Build history of the part. All positions in model axes, mm. Face numbers are marked on the shaded views. Round coordinates to 2 decimals unless told otherwise and drop trailing zeros. Loops run counter-clockwise (first coordinate to the right, second up) from the corner with the lowest first, then second, coordinate; pieces in that order, holes last. Notation, with made-up numbers: M 0,-10.75 L 49,-10.75 A30 cw 49,12.25 Z; hole C 84,82 d7. An arc over 180 degrees is marked long. One line per item, written item: value.
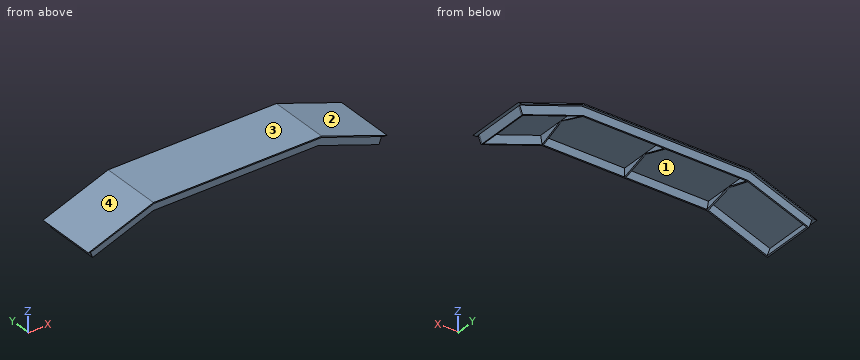
```python
from build123d import *

# Parameters (mm, degrees)
BOSS_EXTRUDE1_DEPTH = 109.600000002
BOSS_EXTRUDE2_DEPTH = 2.54
BOSS_EXTRUDE3_DEPTH = 2.54
RIB2_REACH          = 442.308
SKETCH5_WALL_W      = 932.745237508
SKETCH5_WALL_H      = 2.54
RIB3_REACH          = 442.308
SKETCH6_WALL_W      = 932.745237508
SKETCH6_WALL_H      = 2.54
RIB4_REACH          = 442.308
SKETCH7_WALL_W      = 932.745237508
SKETCH7_WALL_H      = 2.54
RIB5_REACH          = 442.308
SKETCH8_WALL_W      = 932.745237508
SKETCH8_WALL_H      = 2.54
RIB6_REACH          = 332.895
SKETCH13_WALL_W     = 713.849927416
SKETCH13_WALL_H     = 2.54
RIB7_REACH          = 332.895
SKETCH14_WALL_W     = 713.849927416
SKETCH14_WALL_H     = 2.54
SKETCH15_W          = 2.54
SKETCH15_H          = 95.520000222
BOSS_EXTRUDE4_DEPTH = 15
SKETCH16_W          = 2.54
SKETCH16_H          = 95.520000222
BOSS_EXTRUDE5_DEPTH = 15


with BuildPart() as part:
    # Sketch1 → Boss-Extrude1 (new body)
    with BuildSketch(Plane(origin=(0, 0, 0), x_dir=(1, 0, 0), z_dir=(0, 1, 0))):
        Polygon((-261, -120), (-150, -160), (150, -160), (261, -120), (266.899364373, -120), (150.349364373, -162), (-150.349364373, -162), (-266.899364373, -120), align=None)
    extrude(amount=BOSS_EXTRUDE1_DEPTH)

    # Sketch2 → Boss-Extrude2 (add)
    with BuildSketch(Plane(origin=(0, 4.49999989, 0), x_dir=(1, 0, 0), z_dir=(0, 1, 0))):
        Polygon((147.379767206, -145), (255.914706381, -105.888310207), (261, -120), (150, -160), (-150, -160), (-261, -120), (-255.914706381, -105.888310207), (-147.379767206, -145), align=None)
    extrude(amount=BOSS_EXTRUDE2_DEPTH)

    # Sketch4 → Boss-Extrude3 (add)
    with BuildSketch(Plane(origin=(0, 105.100000112, 0), x_dir=(1, 0, 0), z_dir=(0, 1, 0))):
        Polygon((-255.914706381, -105.888310207), (-147.379767206, -145), (147.379767206, -145), (255.914706381, -105.888310207), (261, -120), (150, -160), (-150, -160), (-261, -120), align=None)
    extrude(amount=-BOSS_EXTRUDE3_DEPTH)

    # Sketch5 wall → Rib2 (add, up to next)
    with BuildSketch(Plane(origin=(-148.689883603, 78.680000057, 152.5), x_dir=(-0.052270147277, -0.952748261703, 0.299229980995), z_dir=(0.163945637159, -0.303761007739, -0.938536668561)), mode=Mode.PRIVATE) as rib2_sk1:
        Rectangle(SKETCH5_WALL_W, SKETCH5_WALL_H)
    rib2_tool1 = extrude(rib2_sk1.sketch, amount=-RIB2_REACH, mode=Mode.PRIVATE) - part.part
    add(rib2_tool1.solids().sort_by_distance((-148.689883603, 78.680000057, 152.5))[0])

    # Sketch6 wall → Rib3 (add, up to next)
    with BuildSketch(Plane(origin=(-148.689883603, 30.919999945, 152.5), x_dir=(0.052270147277, -0.952748261703, -0.299229980995), z_dir=(0.163945637159, 0.303761007739, -0.938536668561)), mode=Mode.PRIVATE) as rib3_sk1:
        Rectangle(SKETCH6_WALL_W, SKETCH6_WALL_H)
    rib3_tool1 = extrude(rib3_sk1.sketch, amount=-RIB3_REACH, mode=Mode.PRIVATE) - part.part
    add(rib3_tool1.solids().sort_by_distance((-148.689883603, 30.919999945, 152.5))[0])

    # Sketch7 wall → Rib4 (add, up to next)
    with BuildSketch(Plane(origin=(148.689883603, 78.680000057, 152.5), x_dir=(0.052270147277, -0.952748261703, 0.299229980995), z_dir=(-0.163945637159, -0.303761007739, -0.938536668561)), mode=Mode.PRIVATE) as rib4_sk1:
        Rectangle(SKETCH7_WALL_W, SKETCH7_WALL_H)
    rib4_tool1 = extrude(rib4_sk1.sketch, amount=-RIB4_REACH, mode=Mode.PRIVATE) - part.part
    add(rib4_tool1.solids().sort_by_distance((148.689883603, 78.680000057, 152.5))[0])

    # Sketch8 wall → Rib5 (add, up to next)
    with BuildSketch(Plane(origin=(148.689883603, 30.919999945, 152.5), x_dir=(-0.052270147277, -0.952748261703, -0.299229980995), z_dir=(-0.163945637159, 0.303761007739, -0.938536668561)), mode=Mode.PRIVATE) as rib5_sk1:
        Rectangle(SKETCH8_WALL_W, SKETCH8_WALL_H)
    rib5_tool1 = extrude(rib5_sk1.sketch, amount=-RIB5_REACH, mode=Mode.PRIVATE) - part.part
    add(rib5_tool1.solids().sort_by_distance((148.689883603, 30.919999945, 152.5))[0])

    # Sketch13 wall → Rib6 (add, up to next)
    with BuildSketch(Plane(origin=(0, 78.680000057, 152.5), x_dir=(0, -0.954052469095, 0.299639593869), z_dir=(0, -0.299639593869, -0.954052469095)), mode=Mode.PRIVATE) as rib6_sk1:
        Rectangle(SKETCH13_WALL_W, SKETCH13_WALL_H)
    rib6_tool1 = extrude(rib6_sk1.sketch, amount=-RIB6_REACH, mode=Mode.PRIVATE) - part.part
    add(rib6_tool1.solids().sort_by_distance((0, 78.680000057, 152.5))[0])

    # Sketch14 wall → Rib7 (add, up to next)
    with BuildSketch(Plane(origin=(0, 30.919999945, 152.5), x_dir=(0, -0.954052469095, -0.299639593869), z_dir=(0, 0.299639593869, -0.954052469095)), mode=Mode.PRIVATE) as rib7_sk1:
        Rectangle(SKETCH14_WALL_W, SKETCH14_WALL_H)
    rib7_tool1 = extrude(rib7_sk1.sketch, amount=-RIB7_REACH, mode=Mode.PRIVATE) - part.part
    add(rib7_tool1.solids().sort_by_distance((0, 30.919999945, 152.5))[0])

    # Sketch15 → Boss-Extrude4 (add)
    with BuildSketch(Plane(origin=(68.270957546, 0, 189.451907191), x_dir=(-0.9407793195201408, 0, 0.33901957460185245), z_dir=(-0.3390195746018524, 0, -0.9407793195201407))):
        with Locations((-203.591053443, 54.800000001)):
            Rectangle(SKETCH15_W, SKETCH15_H)
    extrude(amount=BOSS_EXTRUDE4_DEPTH)

    # Sketch16 → Boss-Extrude5 (add)
    with BuildSketch(Plane(origin=(-68.270957546, 0, 189.451907191), x_dir=(-0.9407793195201407, 0, -0.3390195746018526), z_dir=(0.3390195746018526, 0, -0.9407793195201408))):
        with Locations((203.591053443, 54.800000001)):
            Rectangle(SKETCH16_W, SKETCH16_H)
    extrude(amount=BOSS_EXTRUDE5_DEPTH)


solid = part.part
```
Item 1: Drop flat-ended pins along their axis: P1, Ø3, axis at x = 264.5, y = 42.5, coming from the -Z side; P2, Ø7.5, axis at x = 76.5, z = 152, coming from the +Y side; P3, Ø8, axis at y = 26.5, z = 122.5, coming from the +X side. Give the stop position or say it passes through.
Check values:
P1: stops at z = 120
P2: stops at y = 105.1
P3: stops at x = 266.9
Item 2: Pull direction X, two halves, no side cores. Call the marked faces 1, 2, 3 and 4: pulls with the +X half, pulls with the -X half, needs draft (parallel to the pull), parting line crosses it, or undercut.
Check values:
face 1: undercut
face 2: pulls with the +X half
face 3: needs draft
face 4: pulls with the -X half
Item 3: Slice it at C-C, the plane y = 71.5. Give the cut face in (x, z).
Check values:
outline: M -266.9,120 L -261,120 L -255.91,105.89 L -253.53,106.75 L -258.61,120.86 L -151.21,159.56 L -150.33,154.54 L -147.83,154.97 L -148.71,160 L -1.27,160 L -1.27,154.76 L 1.27,154.76 L 1.27,160 L 148.71,160 L 147.83,154.97 L 150.33,154.54 L 151.21,159.56 L 258.61,120.86 L 253.53,106.75 L 255.91,105.89 L 261,120 L 266.9,120 L 150.35,162 L -150.35,162 Z
Item 4: Slice it at A-A, the plane x = 138. Give the cut face in (y, z).
Check values:
outline: M 0,160 L 4.5,160 L 4.5,145 L 7.04,145 L 7.04,160 L 102.56,160 L 102.56,145 L 105.1,145 L 105.1,160 L 109.6,160 L 109.6,162 L 0,162 Z
Item 5: Wall check: line 1 along Y through (x, z) = (-79, 156); line 2 along Z through (x, y) = (60, 40.5); line 3 along X through (y, z) = (93.5, 116). Give the ranges that are in metal, low to high.
Check values:
line 1: y = 4.5 to 7.04, 102.56 to 105.1
line 2: z = 160 to 162
line 3: x = -259.56 to -256.86, 256.86 to 259.56
Item 6: Slice it at B-B, the plane z = 131.5. Give the cut face in (x, y), and give its area (3 significant figures).
Check values:
outline: M -234.99,0 L -229.09,0 L -229.09,4.5 L -184.84,4.5 L -184.84,7.04 L -229.09,7.04 L -229.09,102.56 L -184.84,102.56 L -184.84,105.1 L -229.09,105.1 L -229.09,109.6 L -234.99,109.6 Z; M 184.84,4.5 L 229.09,4.5 L 229.09,0 L 234.99,0 L 234.99,109.6 L 229.09,109.6 L 229.09,105.1 L 184.84,105.1 L 184.84,102.56 L 229.09,102.56 L 229.09,7.04 L 184.84,7.04 Z
area: 1,740 mm2
Item 7: Slice it at D-D, the plane y = 37.5. Give the cut face in (x, z).
Check values:
outline: M -266.9,120 L -261,120 L -255.91,105.89 L -253.53,106.75 L -258.61,120.86 L -151.21,159.56 L -150.3,154.35 L -147.8,154.79 L -148.71,160 L -1.27,160 L -1.27,154.57 L 1.27,154.57 L 1.27,160 L 148.71,160 L 147.8,154.79 L 150.3,154.35 L 151.21,159.56 L 258.61,120.86 L 253.53,106.75 L 255.91,105.89 L 261,120 L 266.9,120 L 150.35,162 L -150.35,162 Z
